Work out the finished part from the listing and answer in its coordinate system (mm). Face numbers are marked on the shaded views. A direction names the side the tool comes from. Give positions to 0.01 mm unless a question says otherwise; leave off trailing zeros. Order: outer loops, then holes, each group sorted by start corner. A loop starts at its lowest first (then second) coordinate and runs counter-clockwise, first axis right, second up. Notation, with made-up numbers: M 61.25,80 L 112.25,80 A6 ccw 112.25,86 Z; hole C 5.5,83.5 d9. An arc over 180 degrees is marked long. One line per item, written item: value.
Autodesk Inventor part; units mm, degrees
ref_plane "YZ Plane" through (0, 0, 0) normal (1, 0, 0) x (0, 1, 0)
ref_plane "XZ Plane" through (0, 0, 0) normal (0, 1, 0) x (-1, 0, 0)
ref_plane "XY Plane" through (0, 0, 0) normal (0, 0, 1) x (1, 0, 0)
sketch "Sketch1" plane through (0, 0, 0) normal (0, 0, 1) x (1, 0, 0)
  line L0 (0, 0) -> (9.2453, 0)
  line L1 (0, 0) -> (177.8, 0)
  line L2 (177.8, 0) -> (177.8, 50.8)
  line L3 (177.8, 50.8) -> (50.8, 50.8)
  line L4 (50.8, 50.8) -> (50.8, 127)
  line L5 (50.8, 127) -> (0, 127)
  line L6 (0, 127) -> (0, 0)
  dimension "d0" = 177.8
  dimension "d1" = 50.8
  dimension "d2" = 127
  dimension "d3" = 76.2
  dimension "d4" = 50.8
extrude "Extrusion1" add sketch "Sketch1" along normal blind 127
sketch "Sketch2" plane through (177.8, 0, 0) normal (1, 0, 0) x (0, 0, -1)
  line L0 (0, 50.8) -> (-127, 50.8)
  line L1 (-63.5, 50.8) -> (-50.8, 50.8)
  line L2 (-50.8, 50.8) -> (-76.2, 50.8)
  line L3 (-76.2, 50.8) -> (-76.2, 0)
  line L4 (-76.2, 0) -> (-50.8, 0)
  line L5 (-50.8, 0) -> (-50.8, 50.8)
  point P0 (0, 0)
  dimension "d7" = 12.7
  dimension "d8" = 25.4
  dimension "d9" = 50.8
extrude "Extrusion2" cut sketch "Sketch2" against normal blind 76.2
sketch "Sketch3" plane through (0, 127, 0) normal (0, 1, 0) x (1, 0, 0)
  line L0 (0, 0) -> (0, -127)
  line L1 (0, -63.5) -> (0, -101.6)
  line L2 (0, -101.6) -> (50.8, -101.6)
  line L3 (50.8, -101.6) -> (50.8, -25.4)
  line L4 (50.8, -25.4) -> (0, -25.4)
  line L5 (0, -25.4) -> (0, -101.6)
  dimension "d12" = 38.1
  dimension "d13" = 50.8
  dimension "d14" = 76.2
extrude "Extrusion3" cut sketch "Sketch3" against normal blind 25.4
properties part number "10-18-19 A"
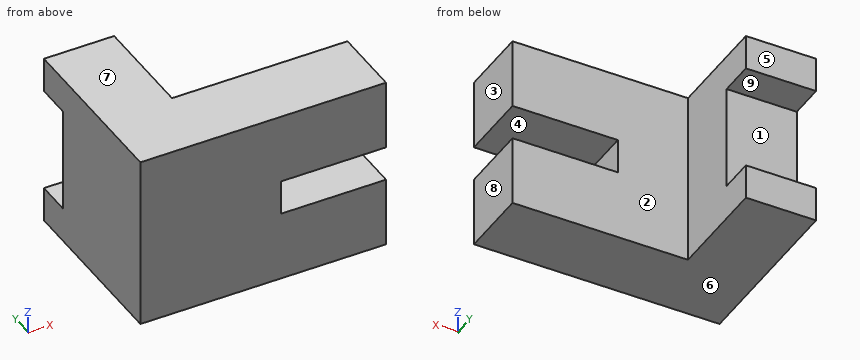
(1) Find the intervals of material crossed by probe 1 along Z at (x, y) = (108, 21); probe 2 along Z at (x, y) = (9.5, 103); probe 3 along X at (y, z) = (59, 94), in increasing order. Write a range as from..to.
Findings:
probe 1: z = 0..50.8, 76.2..127
probe 2: z = 0..25.4, 101.6..127
probe 3: x = 0..50.8
(2) Section A-A, the plane x = 130.5 is taken. Give the vertices of the cut face in (y, z).
Findings:
outline: M 0,0 L 50.8,0 L 50.8,50.8 L 0,50.8 Z; M 0,76.2 L 50.8,76.2 L 50.8,127 L 0,127 Z
(3) Section D-D, the plane x = 25.5 is taken. Give the vertices of the cut face in (y, z).
Findings:
outline: M 0,0 L 127,0 L 127,25.4 L 101.6,25.4 L 101.6,101.6 L 127,101.6 L 127,127 L 0,127 Z
(4) Determine the mould class of the marked faces 6, 7, 8 and 9 for opening direction Z: pulls with the +Z half, pulls with the -Z half, needs draft (parallel to the pull), parting line crosses it, or undercut.
Findings:
face 6: pulls with the -Z half
face 7: pulls with the +Z half
face 8: needs draft
face 9: undercut
(5) Section B-B, the plane y = 104 is taken. Give the vertices of the cut face in (x, z).
Findings:
outline: M 0,0 L 50.8,0 L 50.8,25.4 L 0,25.4 Z; M 0,101.6 L 50.8,101.6 L 50.8,127 L 0,127 Z
(6) Given P1, Ø23, axis at y = 77, z = 70.5, coming from the +X side, flat-ended and moving along its own axis, determine where the tip first touches the part or whether it passes through.
Findings:
P1: stops at x = 50.8
(7) Section C-C, the plane z = 37 is taken. Give the vertices of the cut face in (x, y), then the cut area to 3 significant figures.
Findings:
outline: M 0,0 L 177.8,0 L 177.8,50.8 L 50.8,50.8 L 50.8,101.6 L 0,101.6 Z
area: 11,600 mm^2
(8) Which of the six approach directions +Z, -Z, +X, -X, +Y, -Y give full straight-line access (tool end or side, diameter ignored) to the marked faces 1, 2, 3, 4 and 5?
Findings:
face 1: +X, -X, +Y
face 2: +Z, -Z, +X, +Y
face 3: +Z, -Z, +X, +Y, -Y
face 4: +X, +Y, -Y
face 5: +Z, -Z, +X, -X, +Y
